from build123d import *

# Parameters (mm, degrees)
SKETCH1_W             = 50
SKETCH1_H             = 50
BOSS_EXTRUDE1_DEPTH   = 25
BOSS_EXTRUDE2_DEPTH   = 22.5
SKETCH4_W             = 80
SKETCH4_H             = 90
BOSS_EXTRUDE4_DEPTH   = 30
SKETCH5_W             = 25
SKETCH5_H             = 25
BOSS_EXTRUDE5_DEPTH   = 10
SKETCH6_W             = 25
SKETCH6_H             = 60
BOSS_EXTRUDE6_DEPTH   = 10
SKETCH7_W             = 15
SKETCH7_H             = 10
BOSS_EXTRUDE7_DEPTH   = 50
SKETCH8_W             = 19
SKETCH8_H             = 30
BOSS_EXTRUDE10_DEPTH  = 5
MIRROR3_START         = -1.25
MIRROR3_DEPTH         = 15
MIRROR3_START_2       = 36.25
MIRROR3_2_OUTLINE_W   = 5
MIRROR3_2_OUTLINE_H   = 2
MIRROR3_2_OUTLINE_W_2 = 50
MIRROR3_2_OUTLINE_H_2 = 10
MIRROR3_2_DEPTH       = 15
MIRROR3_START_3       = -3.25
MIRROR3_3_OUTLINE_W   = 5
MIRROR3_3_OUTLINE_H   = 32
MIRROR3_3_DEPTH       = 19
MIRROR3_START_4       = 34.25
MIRROR3_4_OUTLINE_W   = 5
MIRROR3_4_OUTLINE_H   = 2
MIRROR3_4_DEPTH       = 19
SKETCH9_W             = 74.5
SKETCH9_H             = 44
BOSS_EXTRUDE11_DEPTH  = 5
SKETCH10_R            = 17.5
CUT_EXTRUDE1_DEPTH    = 10


# Read off the part's stored shape, not the designer's step: Mirror3
with BuildPart() as part:
    # Sketch1 → Boss-Extrude1 (new, symmetric)
    with BuildSketch(Plane.XY):
        with Locations((25, 25)):
            Rectangle(SKETCH1_W, SKETCH1_H)
    extrude(amount=BOSS_EXTRUDE1_DEPTH, both=True)

    # Sketch2 → Boss-Extrude2 (add, symmetric)
    with BuildSketch(Plane.XY):
        Polygon((0, 50), (24.011645754, 90), (50, 50), align=None)
    extrude(amount=BOSS_EXTRUDE2_DEPTH, both=True)

    # Sketch4 → Boss-Extrude4 (add, symmetric)
    with BuildSketch(Plane.XY):
        with Locations((25, -45)):
            Rectangle(SKETCH4_W, SKETCH4_H)
    extrude(amount=BOSS_EXTRUDE4_DEPTH, both=True)

    # Sketch5 → Boss-Extrude5 (add)
    with BuildSketch(Plane(origin=(65, 0, 0), x_dir=(0, 0, -1), z_dir=(1, 0, 0))):
        with Locations((5, -37.5)):
            Rectangle(SKETCH5_W, SKETCH5_H)
    boss_extrude5 = extrude(amount=BOSS_EXTRUDE5_DEPTH)

    # Sketch6 → Boss-Extrude6 (add)
    with BuildSketch(Plane(origin=(75, 0, 0), x_dir=(0, 0, -1), z_dir=(1, 0, 0))):
        with Locations((5, -55)):
            Rectangle(SKETCH6_W, SKETCH6_H)
    boss_extrude6 = extrude(amount=BOSS_EXTRUDE6_DEPTH)

    # Mirror1: Boss-Extrude5, Boss-Extrude6 across plane
    add(boss_extrude5.mirror(Plane(origin=(25, 0, 0), x_dir=(0, 0, 1), z_dir=(1, 0, 0))))
    add(boss_extrude6.mirror(Plane(origin=(25, 0, 0), x_dir=(0, 0, 1), z_dir=(1, 0, 0))))

    # Sketch7 → Boss-Extrude7 (add)
    with BuildSketch(Plane.XZ.offset(90)):
        with Locations((43.75, -0.5)):
            Rectangle(SKETCH7_W, SKETCH7_H)
    extrude(amount=BOSS_EXTRUDE7_DEPTH)

    # Sketch8 → Boss-Extrude10 (add)
    with BuildSketch(Plane.XZ.offset(140)):
        with Locations((43.75, 5.5)):
            Rectangle(SKETCH8_W, SKETCH8_H)
    extrude(amount=BOSS_EXTRUDE10_DEPTH)

    # Mirror3 outline → Mirror3 (add)
    with BuildSketch(Plane.YZ.offset(MIRROR3_START)):
        Polygon((-90, -5.5), (-90, 14.5), (-140, 14.5), (-140, 20.5), (-145, 20.5), (-145, -11.5), (-140, -11.5), (-140, -5.5), align=None)
    extrude(amount=MIRROR3_DEPTH)

    # Mirror3 2 outline → Mirror3 2 (add)
    with BuildSketch(Plane.YZ.offset(MIRROR3_START_2)):
        with Locations((-142.5, -10.5)):
            Rectangle(MIRROR3_2_OUTLINE_W, MIRROR3_2_OUTLINE_H)
        with Locations((-115, 9.5)):
            Rectangle(MIRROR3_2_OUTLINE_W_2, MIRROR3_2_OUTLINE_H_2)
    extrude(amount=MIRROR3_2_DEPTH)

    # Mirror3 3 outline → Mirror3 3 (add)
    with BuildSketch(Plane.YZ.offset(MIRROR3_START_3)):
        with Locations((-142.5, 4.5)):
            Rectangle(MIRROR3_3_OUTLINE_W, MIRROR3_3_OUTLINE_H)
    extrude(amount=MIRROR3_3_DEPTH)

    # Mirror3 4 outline → Mirror3 4 (add)
    with BuildSketch(Plane.YZ.offset(MIRROR3_START_4)):
        with Locations((-142.5, -10.5)):
            Rectangle(MIRROR3_4_OUTLINE_W, MIRROR3_4_OUTLINE_H)
    extrude(amount=MIRROR3_4_DEPTH)

    # Sketch9 → Boss-Extrude11 (add)
    with BuildSketch(Plane.XZ.offset(145)):
        with Locations((25, 4.5)):
            Rectangle(SKETCH9_W, SKETCH9_H)
    extrude(amount=BOSS_EXTRUDE11_DEPTH)

    # Sketch10 → Cut-Extrude1 (cut)
    with BuildSketch(Plane.XY.offset(25)):
        with Locations((25, 25)):
            Circle(SKETCH10_R)
    extrude(amount=-CUT_EXTRUDE1_DEPTH, mode=Mode.SUBTRACT)


solid = part.part
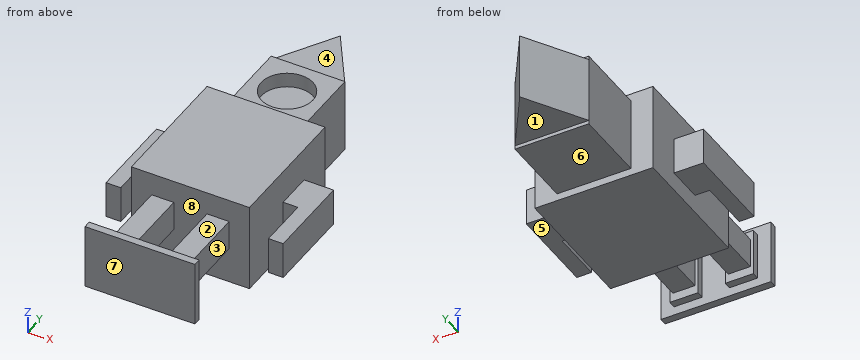
For this review, take the finished solid that the model builds, in its own axes (mm). Face numbers are marked on the shaded views. A direction names the side the tool comes from. Give positions to 0.01 mm unless a question says otherwise; leave off trailing zeros. Order: outer loops, then holes, each group sorted by start corner. A loop starts at its lowest first (then second) coordinate and runs counter-clockwise, first axis right, second up. Notation, with made-up numbers: (20.25, 6) - (78.25, 6) arc R21 cw to (78.25, 32) - close; hole circle Ø3 at (84, 35). An arc over 180 degrees is marked (long way). Answer as a JSON object with one key per item and string values. Group by question number.
Item 1: Machinability: for the marked faces 1, 2, 3, 4 and 5, which of the approach directions +Z, -Z, +X, -X, +Y, -Y give a long, thin tool a straight path to every point of the face, cutting with its end or side? Answer none if there is none.
Item 2: Wall thickness on line 1 along Y through (x, z) = (60.5, -2.5); line 2 along Z through (x, y) = (-18, -49.5); line 3 along X through (y, z) = (46, 6): over which ranges is each line inside the solid? List them lowest first.
Item 3: Draft analysis for pull direction Y (two halves, no side actions). For the marked faces 6, 7 and 8, state which applies: pulls with the +Y half, pulls with the -Y half, needs draft (parallel to the pull), parting line crosses it, or undercut.
Item 4: Take a section at A-A on y = -129. Give the boundary of the cut face in (x, z), and give its area (3 significant figures).
Item 5: Take a section at C-C on y = 25. Give the boundary of the cut face in (x, z).
Item 6: Take a section at D-D on x = 21. Give the boundary of the cut face in (y, z), and give its area (3 significant figures).
Item 7: Clearance check with flat-ended pins moving along their axes: pin 1 Ø22 at (x, z) = (74, -5.5) entering from +Y; pin 2 Ø4 at (x, z) = (67.5, 2) entering from +Y; pin 3 Ø10 at (x, y) = (-21, -48) entering from -Z. State where each tip first meets the part, or that it passes through.
Item 8: Take a section at B-B on x = 55.5. Give the boundary of the cut face in (y, z), and give its area (3 significant figures).
Reported:
{
 "1": {"face 1": "-Z, +X, -X, +Y", "face 2": "+Z, +X, -X", "face 3": "+Z, -Z, +X", "face 4": "+Z, +X, -X, +Y", "face 5": "-Z, +X, +Y, -Y"},
 "2": {"line 1": "-150 to -145, -90 to 0", "line 2": "-17.5 to 7.5", "line 3": "0 to 50"},
 "3": {"face 6": "needs draft", "face 7": "pulls with the -Y half", "face 8": "undercut"},
 "4": {"outline": "(-1.25, -5.5) - (13.75, -5.5) - (13.75, 14.5) - (-1.25, 14.5) - close; (36.25, -5.5) - (51.25, -5.5) - (51.25, 14.5) - (36.25, 14.5) - close", "area": "600 mm^2"},
 "5": {"outline": "(0, -25) - (50, -25) - (50, 25) - (42.5, 25) - (42.5, 15) - (7.5, 15) - (7.5, 25) - (0, 25) - close"},
 "6": {"outline": "(-150, -17.5) - (-145, -17.5) - (-145, 26.5) - (-150, 26.5) - close; (-90, -30) - (0, -30) - (0, -25) - (50, -25) - (50, -22.5) - (84.98, -22.5) - (84.98, 22.5) - (50, 22.5) - (50, 25) - (42.04, 25) - (42.04, 15) - (7.96, 15) - (7.96, 25) - (0, 25) - (0, 30) - (-90, 30) - close", "area": "9,350 mm^2"},
 "7": {"pin 1": "y = 0", "pin 2": "y = -25", "pin 3": "z = -17.5"},
 "8": {"outline": "(-150, -17.5) - (-145, -17.5) - (-145, 26.5) - (-150, 26.5) - close; (-90, -30) - (0, -30) - (0, 30) - (-90, 30) - close", "area": "5,620 mm^2"}
}
